```python
from build123d import *

# Parameters (mm, degrees)
F0_W     = 94.059766
F0_H     = 100.90065
F1_DEPTH = 4
F6_W     = 72.467298
F6_H     = 61.010792
F2_DEPTH = 25
F3_W     = 7.757127
F3_H     = 6.220043
F4_DEPTH = 25
F5_R     = 2


with BuildPart() as f1:
    # F0 (on Top) → F1 (new body)
    with BuildSketch(Plane.XY):
        Rectangle(F0_W, F0_H)
    extrude(amount=F1_DEPTH)

    # F6 (on face) → F2 (cut)
    with BuildSketch(Plane.XY.offset(4)):
        Rectangle(F6_W, F6_H)
    extrude(amount=-F2_DEPTH, mode=Mode.SUBTRACT)

    # F3 (on face) → F4 (cut)
    with BuildSketch(Plane.XY.offset(4)):
        with Locations((-20.997285, -39.404213)):
            Rectangle(F3_W, F3_H)
    extrude(amount=-F4_DEPTH, mode=Mode.SUBTRACT)

    # F5
    f5_edges = [f1.edges().sort_by_distance(p)[0] for p in [
        (-24.875849, -36.294192, 2),
        (-24.875849, -42.514235, 2),
        (-17.118722, -42.514235, 2),
        (-17.118722, -36.294192, 2),
    ]]
    fillet(f5_edges, radius=F5_R)


solid = f1.part
```
Verification items for the finished model (mm, model axes). A direction names the side the tool comes from. Round coordinates to 2 decimals unless told otherwise and drop trailing zeros. Order: outer loops, then holes, each group sorted by start corner. A loop starts at its lowest first (then second) coordinate and runs counter-clockwise, first axis right, second up.
1) Draft check along X on faces 3 (the flat face through (-1, 50.45, 2)), 4 (the flat face through (-47.03, -1, 2)), 5 (the flat face through (36.234, 0, 2)). Enter one of: +X half, -X half, draft (parallel to the pull), parting line (faces both ways), or undercut.
Geometry says:
face 3: draft
face 4: -X half
face 5: undercut
2) Material ranges on line 1 (X direction, y = 18, z = 0.2); line 2 (Y direction, x = -6, z = 1.9); line 3 (X direction, y = -39.5, z = 0.5), recorded low to high.
Geometry says:
line 1: x = -47.03 to -36.23, 36.23 to 47.03
line 2: y = -50.45 to -30.51, 30.51 to 50.45
line 3: x = -47.03 to -24.88, -17.12 to 47.03
3) Cross-section at D-D, the plane x = -21.5. Record the cut outline in (y, z).
Geometry says:
outline: (-50.45, 0) - (-42.51, 0) - (-42.51, 4) - (-50.45, 4) - close; (-36.29, 0) - (-30.51, 0) - (-30.51, 4) - (-36.29, 4) - close; (30.51, 0) - (50.45, 0) - (50.45, 4) - (30.51, 4) - close
4) Cross-section at A-A, the plane x = -4. Record the cut outline in (y, z).
Geometry says:
outline: (-50.45, 0) - (-30.51, 0) - (-30.51, 4) - (-50.45, 4) - close; (30.51, 0) - (50.45, 0) - (50.45, 4) - (30.51, 4) - close
5) Tool access check on faces 1 (the flat face through (-24.876, -39, 2)), 2 (the flat face through (47.03, -1, 2)). Record the directions out of +Z, -Z, +X, -X, +Y, -Y that give a thin tool (end or side, any length) a straight path to the whole face; none if there is none.
Geometry says:
face 1: +Z, -Z
face 2: +Z, -Z, +X, +Y, -Y
6) Cross-section at C-C, the plane z = 1.05. Record the cut outline in (x, y).
Geometry says:
outline: (-47.03, -50.45) - (47.03, -50.45) - (47.03, 50.45) - (-47.03, 50.45) - close; hole (-36.23, -30.51) - (36.23, -30.51) - (36.23, 30.51) - (-36.23, 30.51) - close; hole (-24.88, -40.51) arc R2 ccw to (-22.88, -42.51) - (-19.12, -42.51) arc R2 ccw to (-17.12, -40.51) - (-17.12, -38.29) arc R2 ccw to (-19.12, -36.29) - (-22.88, -36.29) arc R2 ccw to (-24.88, -38.29) - close
7) Cross-section at B-B, the plane y = -9.5. Record the cut outline in (x, z), plus the area to 3 significant figures.
Geometry says:
outline: (-47.03, 0) - (-36.23, 0) - (-36.23, 4) - (-47.03, 4) - close; (36.23, 0) - (47.03, 0) - (47.03, 4) - (36.23, 4) - close
area: 86.4 mm2
